Design review of the part shown in the three views and the two pictorial views. Dimensions are in mm from the part's minimum x, y and z. A direction names the side the tool comes from. Coordinates: 2 decimals unless noted, no trailing zeros. Order: outer loops, then holes, each group sorted by start corner. A loop starts at its lowest first (then second) coordinate and runs counter-clockwise, first axis right, second up. Notation, with made-up numbers: (24, 15) - (32, 15) arc R31 cw to (32, 49) - close; hole circle Ø11 at (10.5, 84). An arc over 180 degrees is marked (long way). One line per item, written item: value. Start each with the question number.
(1) Mouldability with a two-part tool opening along X and no side actions: class the marked faces 1, 2 and 3 as released by +X, released by -X, zero draft, split by the parting line, or undercut.
(2) For the marked faces 4, 5 and 6, list the 3-axis set-ups (+Z, -Z, +X, -X, +Y, -Y) from which the entire face can be reached by the end or side of a thin tool; tool diameter is ignored.
(3) Consider section B-B on z = 8.75. Count the separate pieces of the cut face and the enclosed holes in it, then the cut area to 3 significant figures.
(4) Clearance check with flat-ended pins moving along their axes: pin 1 (1 mm diameter, centred on x = 23.5, y = 40, fed in from -Z); pin 2 (16 mm diameter, centred on x = 18.5, y = 52.5, fed in from +Z); pin 3 (1.5 mm diameter, centred on x = 26.5, z = 3, fed in from +Y). State where each tip first meets the part, or that it passes through.
(5) To check wall thickness, follow line 1 along X through (y, z) = (68, 13.5); line 2 along Z through (x, y) = (32, 77). State the ranges of each line that lie inside material, in increasing order.
(6) Consider section D-D on x = 19. Write out the cut boundary in (y, z).
(7) Consider section A-A on y = 16. Write out the cut boundary in (x, z), then the cut area to 3 significant figures.
(8) Consider section C-C on y = 79. Write out the cut boundary in (x, z).
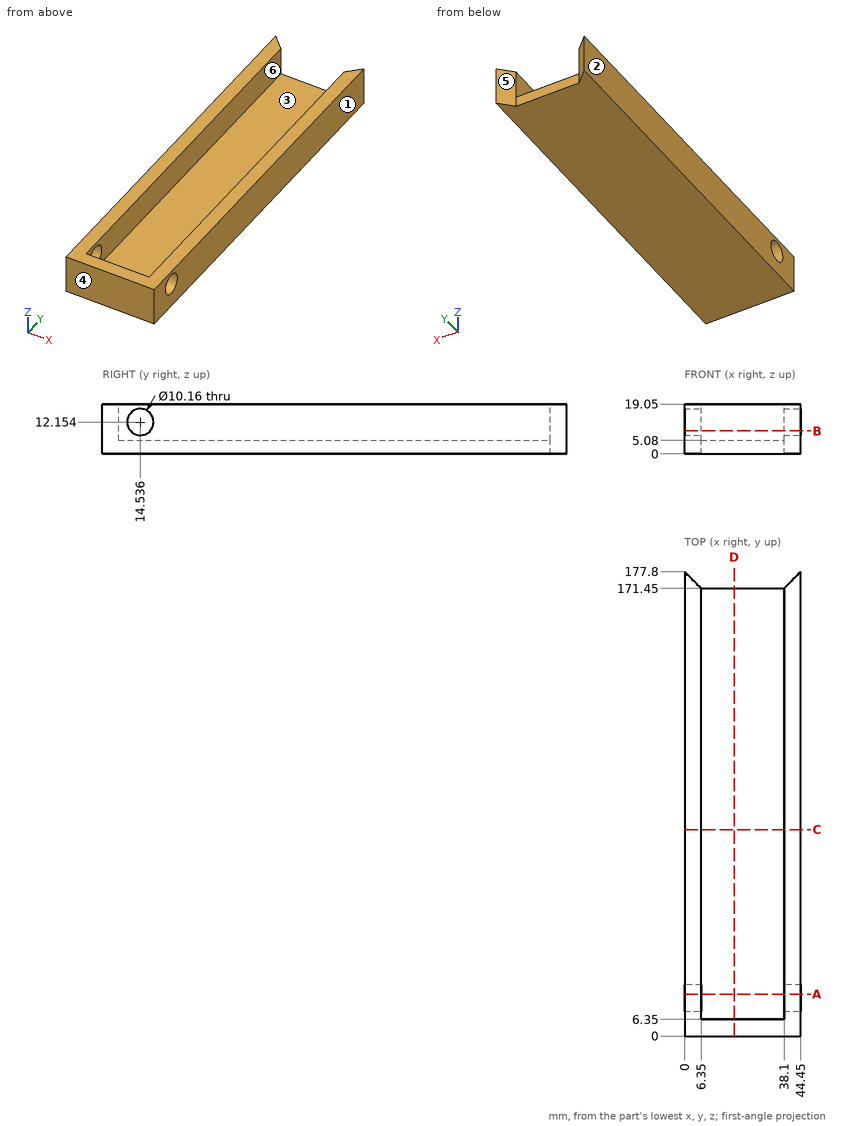
Geometry check:
1. face 1: released by +X
1. face 2: released by -X
1. face 3: undercut
2. face 4: +Z, -Z, +X, -X, -Y
2. face 5: +Z, -Z, +Y
2. face 6: +Z, +Y
3. separate pieces: 3
3. enclosed holes: 0
3. area: 2,320 mm^2
4. pin 1: stops at z = 0
4. pin 2: stops at z = 5.08
4. pin 3: stops at y = 171.45
5. line 1: x = 0 to 6.35, 38.1 to 44.45
5. line 2: z = 0 to 5.08
6. outline: (0, 0) - (171.45, 0) - (171.45, 5.08) - (6.35, 5.08) - (6.35, 19.05) - (0, 19.05) - close
7. outline: (0, 0) - (44.45, 0) - (44.45, 7.29) - (38.1, 7.29) - (38.1, 5.08) - (6.35, 5.08) - (6.35, 7.29) - (0, 7.29) - close; (0, 17.02) - (6.35, 17.02) - (6.35, 19.05) - (0, 19.05) - close; (38.1, 17.02) - (44.45, 17.02) - (44.45, 19.05) - (38.1, 19.05) - close
7. area: 280 mm^2
8. outline: (0, 0) - (44.45, 0) - (44.45, 19.05) - (38.1, 19.05) - (38.1, 5.08) - (6.35, 5.08) - (6.35, 19.05) - (0, 19.05) - close
